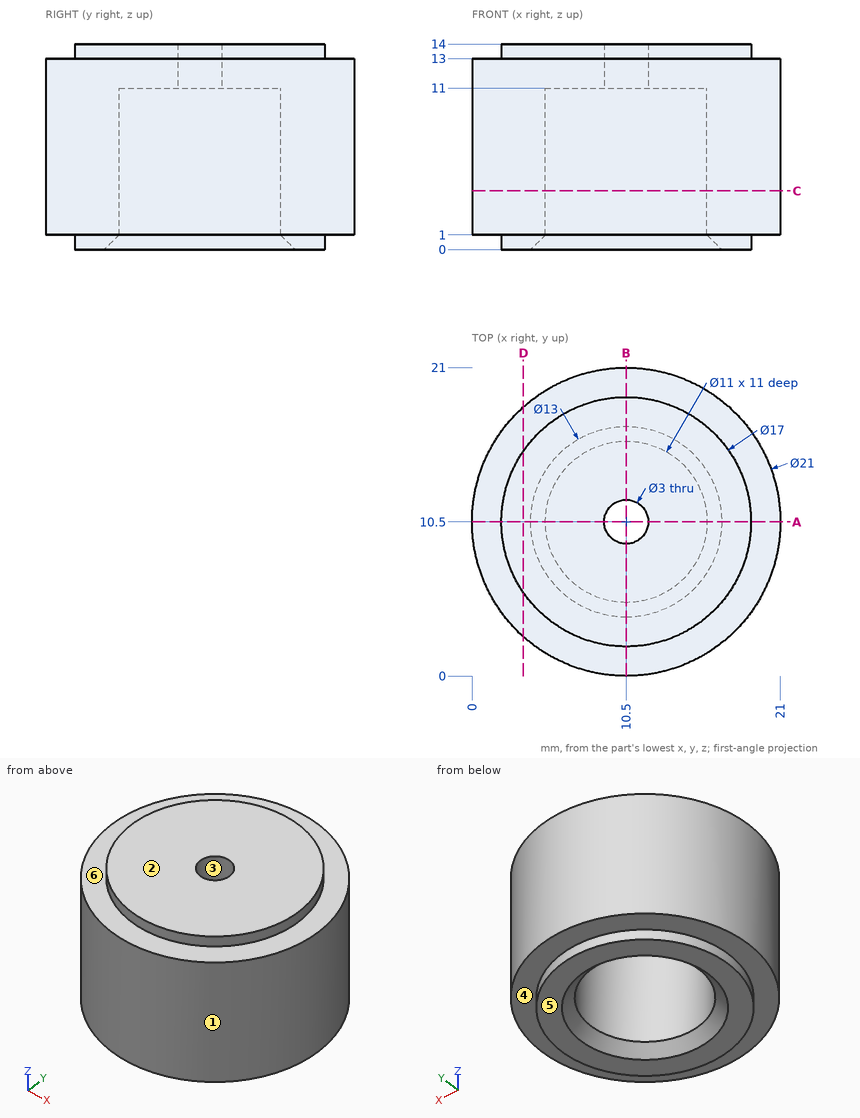
Input: dimensioned drawing with shaded views. Units: mm. Origin: part minimum x, y, z. A direction names the side the tool comes from. Give positions to 0.01 mm unless a question says otherwise; leave off trailing zeros. Write each loop counter-clockwise with the first axis right and the second up, starting at its lowest first coordinate (ties: lowest second). Pieces come first, ordered by that corner, then holes.
1. Section query D-D, the plane x = 3.5. Return loops of the section in (y, z), then the cut area to 3 significant figures.
2. Reachability of the marked faces 4, 5 and 6 from +Z, -Z, +X, -X, +Y, -Y: full face, straight path, thin tool, end or side. Return the list, or none.
3. Section query A-A, the plane y = 10.5. Return loops of the section in (x, z).
4. Pin query (flat end, axial travel): P1, Ø4, axis at x = 2, z = 6, coming from the -Y side; P2, Ø1.5, axis at x = 8, z = 2, coming from the -Y side; P3, Ø6, axis at x = 5.5, z = 10.5, coming from the +Y side; P4, Ø6.5, axis at x = 5.5, y = 7, coming from the -Z side. Return the tip coordinate at first contact, or that it passes through.
5. Line query: probe 1 along X at (y, z) = (10.5, 5.5); probe 2 along Z at (x, y) = (4, 4); probe 3 along Z at (x, y) = (13.75, 14.5). Output: solid intervals per line, ascending.
6. Draft query along X for the marked faces 1, 2 and 3. Return one class per face: released by +X, released by -X, zero draft, split by the parting line, or undercut.
7. Section query C-C, the plane z = 4. Return loops of the section in (x, y), then the cut area to 3 significant figures.
Computed:
1. outline: (2.67, 1) - (5.68, 1) - (5.68, 0) - (15.32, 0) - (15.32, 1) - (18.33, 1) - (18.33, 13) - (15.32, 13) - (15.32, 14) - (5.68, 14) - (5.68, 13) - (2.67, 13) - close
1. area: 207 mm2
2. face 4: -Z
2. face 5: -Z, +X, -X, +Y, -Y
2. face 6: +Z
3. outline: (0, 1) - (2, 1) - (2, 0) - (4, 0) - (5, 1) - (5, 11) - (9, 11) - (9, 14) - (2, 14) - (2, 13) - (0, 13) - close; (12, 11) - (16, 11) - (16, 1) - (17, 0) - (19, 0) - (19, 1) - (21, 1) - (21, 13) - (19, 13) - (19, 14) - (12, 14) - close
4. P1: stops at y = 2.25
4. P2: stops at y = 0.15
4. P3: stops at y = 20.81
4. P4: stops at z = 0
5. probe 1: x = 0 to 5, 16 to 21
5. probe 2: z = 1 to 13
5. probe 3: z = 11 to 14
6. face 1: split by the parting line
6. face 2: zero draft
6. face 3: undercut
7. outline: circle Ø21 at (10.5, 10.5); hole circle Ø11 at (10.5, 10.5)
7. area: 251 mm2
